from build123d import *

# Parameters (mm, degrees)
SKETCH_1_R          = 6
EXTRUDE_1_DEPTH     = 7.5
CUT_EXTRUDE_1_DEPTH = 26.75
SKETCH_4_W          = 4.5
SKETCH_4_H          = 2
CUT_EXTRUDE_2_DEPTH = 7
SKETCH_5_R          = 10
SKETCH_5_R_2        = 6
EXTRUDE_2_DEPTH     = 10
CHAMFER_1_SIZE      = 4
CHAMFER_2_SIZE      = 1
SKETCH_6_R          = 1.5
CUT_EXTRUDE_3_DEPTH = 61.309617807
SKETCH_8_R          = 2.5
CUT_EXTRUDE_4_DEPTH = 8
EXTRUDE_START       = 4
SKETCH_9_R          = 6
SKETCH_9_R_2        = 2.5
EXTRUDE_3_DEPTH     = 4
CHAMFER_4_SIZE      = 2


with BuildPart() as part:
    # 草图1 → 凸台-拉伸1 (new, symmetric)
    with BuildSketch(Plane.XY):
        with BuildLine():
            Line((-42.5, 16), (42.5, 16))
            ThreePointArc((42.5, 16), (49.571067812, 13.071067812), (52.5, 6))
            Line((52.5, 6), (52.5, -6))
            ThreePointArc((52.5, -6), (49.571067812, -13.071067812), (42.5, -16))
            Line((42.5, -16), (-42.5, -16))
            ThreePointArc((-42.5, -16), (-49.571067812, -13.071067812), (-52.5, -6))
            Line((-52.5, -6), (-52.5, 6))
            ThreePointArc((-52.5, 6), (-49.571067812, 13.071067812), (-42.5, 16))
        make_face()
        with Locations((-37.5, 0)):
            Circle(SKETCH_1_R, mode=Mode.SUBTRACT)
        with Locations((37.5, 0)):
            Circle(SKETCH_1_R, mode=Mode.SUBTRACT)
    extrude(amount=EXTRUDE_1_DEPTH, both=True)

    # 草图2 → 切除-拉伸1 (cut)
    with BuildSketch(Plane(origin=(0, 16, 0), x_dir=(1, 0, 0), z_dir=(0, 1, 0))):
        Polygon((13.15, 7.5), (11.35, 7.5), (11.35, 6.52), (9.29, 6.52), (9.29, 3.47), (11.35, 3.47), (11.35, 1.52), (9.29, 1.52), (9.29, -1.53), (11.35, -1.53), (11.35, -3.48), (9.29, -3.48), (9.29, -6.53), (11.35, -6.53), (11.35, -7.5), (13.15, -7.5), align=None)
    extrude(amount=-CUT_EXTRUDE_1_DEPTH, mode=Mode.SUBTRACT)

    # 草图4 → 切除-拉伸2 (cut)
    with BuildSketch(Plane(origin=(0, 16, 0), x_dir=(1, 0, 0), z_dir=(0, 1, 0))):
        with Locations((4.04, 4)):
            Rectangle(SKETCH_4_W, SKETCH_4_H)
        with Locations((4.04, 0)):
            Rectangle(SKETCH_4_W, SKETCH_4_H)
        with Locations((4.04, -4)):
            Rectangle(SKETCH_4_W, SKETCH_4_H)
        with Locations((18.4, 4)):
            Rectangle(SKETCH_4_W, SKETCH_4_H)
        with Locations((18.4, 0)):
            Rectangle(SKETCH_4_W, SKETCH_4_H)
        with Locations((18.4, -4)):
            Rectangle(SKETCH_4_W, SKETCH_4_H)
    extrude(amount=-CUT_EXTRUDE_2_DEPTH, mode=Mode.SUBTRACT)

    # 草图5 → 凸台-拉伸2 (add)
    # profile 1 of 2: a face of its own
    with BuildSketch(Plane.XY.offset(7.5)):
        with Locations(Location((-37.5, 0, 0), (0, 0, 180))):
            Circle(SKETCH_5_R)
        with Locations((-37.5, 0)):
            Circle(SKETCH_5_R_2, mode=Mode.SUBTRACT)
    # profile 2 of 2: a face of its own
    with BuildSketch(Plane.XY.offset(7.5)):
        with Locations(Location((37.5, 0, 0), (0, 0, 180))):
            Circle(SKETCH_5_R)
        with Locations((37.5, 0)):
            Circle(SKETCH_5_R_2, mode=Mode.SUBTRACT)
    extrude(amount=EXTRUDE_2_DEPTH)

    # 倒角1
    chamfer_1_edges = [part.edges().sort_by_distance(p)[0] for p in [
        (-27.5, 0, 7.5),
        (47.5, 0, 7.5),
    ]]
    chamfer(chamfer_1_edges, length=CHAMFER_1_SIZE)

    # 倒角2
    chamfer_2_edges = [part.edges().sort_by_distance(p)[0] for p in [
        (-43.5, 0, 17.5),
        (31.5, 0, 17.5),
    ]]
    chamfer(chamfer_2_edges, length=CHAMFER_2_SIZE)

    # 草图6 → 切除-拉伸3 (cut, through all)
    with BuildSketch(Plane(origin=(0, 0, -7.5), x_dir=(-1, 0, 0), z_dir=(0, 0, -1))):
        with Locations((0, 7.5)):
            Circle(SKETCH_6_R)
        with Locations((0, -7.5)):
            Circle(SKETCH_6_R)
    extrude(amount=-CUT_EXTRUDE_3_DEPTH, mode=Mode.SUBTRACT)

    # 草图8 → 切除-拉伸4 (cut)
    with BuildSketch(Plane.XY.offset(7.5)):
        with Locations((0, 7.5)):
            Circle(SKETCH_8_R)
        with Locations((0, -7.5)):
            Circle(SKETCH_8_R)
    extrude(amount=-CUT_EXTRUDE_4_DEPTH, mode=Mode.SUBTRACT)

    # 草图9 → 凸台-拉伸3 (add)
    # profile 1 of 2: a face of its own
    with BuildSketch(Plane.XY.offset(7.5).offset(EXTRUDE_START)):
        with Locations(Location((0, 7.5, 0), (0, 0, 180))):
            Circle(SKETCH_9_R)
        with Locations((0, 7.5)):
            Circle(SKETCH_9_R_2, mode=Mode.SUBTRACT)
    # profile 2 of 2: a face of its own
    with BuildSketch(Plane.XY.offset(7.5).offset(EXTRUDE_START)):
        with Locations(Location((0, -7.5, 0), (0, 0, 180))):
            Circle(SKETCH_9_R)
        with Locations((0, -7.5)):
            Circle(SKETCH_9_R_2, mode=Mode.SUBTRACT)
    extrude(amount=-EXTRUDE_3_DEPTH)

    # 倒角4
    chamfer_4_edges = [part.edges().sort_by_distance(p)[0] for p in [
        (6, 7.5, 11.5),
        (6, -7.5, 11.5),
    ]]
    chamfer(chamfer_4_edges, length=CHAMFER_4_SIZE)


solid = part.part
Model file for the job. Use its own axes, mm. A direction names the side the tool comes from. Give positions to 0.01 mm unless a question says otherwise; leave off trailing zeros. Loops run counter-clockwise (first coordinate to the right, second up) from the corner with the lowest first, then second, coordinate; pieces in that order, holes last.
1) Flat gauge pins, fed straight in: pin 1 Ø1.6 at (y, z) = (8.5, -3) entering from +X; pin 2 Ø2 at (x, z) = (5, -0.5) entering from +Y; pin 3 Ø6 at (x, z) = (40.5, 11.5) entering from +Y; pin 4 Ø1 at (y, z) = (-11, -0.5) entering from -X. Where does each tip first touch, or does it go through?
2) Tool access for faces 1 (the cylindrical face through (-0.54, -9.94, 5.58)), 2 (the flat face through (18, 13, -3)), 3 (the flat face through (-40, -7, 17.5)): list every direction of +Z, -Z, +X, -X, +Y, -Y with a clear straight run to the whole face (end or side of a thin tool).
3) Saw through at C-C (z = 14.5). Write the cut outline in (x, y).
4) Wall check: line 1 (Z direction, x = 18, y = 12); line 2 (Y direction, x = 0, z = 5.75); line 3 (Y direction, x = 0, z = -5.25). Give the ranges that are in metal, low to high.
5) Saw through at B-B (x = -37.5). Write the cut outline in (y, z), plus the area to 3 significant figures.
6) Pull direction Z, two halves, no side cores. Call faces 4 (the conical face through (-44, 0, 17)), 5 (the flat face through (16.15, 13, -4)), 6 (the flat face through (13.15, 3, 0)): +Z half, -Z half, draft (parallel to the pull), parting line (faces both ways), or undercut.
7) Saw through at A-A (x = 0). Count the separate pieces of the cut face and the enclosed holes in it, plus the area to 3 significant figures.
Answer block:
1. pin 1: stops at x = 52.35
1. pin 2: stops at y = 16
1. pin 3: stops at y = 12.72
1. pin 4: stops at x = -51.43
2. face 1: +Z
2. face 2: +Y
2. face 3: +Z, +X, -X, +Y, -Y
3. outline: circle Ø20 at (-37.5, 0); circle Ø20 at (37.5, 0); hole circle Ø12 at (-37.5, 0); hole circle Ø12 at (37.5, 0)
4. line 1: z = -7.5 to -5, -3 to -1, 1 to 3, 5 to 7.5
4. line 2: y = -16 to -10, -5 to 5, 10 to 16
4. line 3: y = -16 to -9, -6 to 6, 9 to 16
5. outline: (-16, -7.5) - (-6, -7.5) - (-6, 16.5) - (-7, 17.5) - (-10, 17.5) - (-10, 11.5) - (-14, 7.5) - (-16, 7.5) - close; (6, -7.5) - (16, -7.5) - (16, 7.5) - (14, 7.5) - (10, 11.5) - (10, 17.5) - (7, 17.5) - (6, 16.5) - close
5. area: 395 mm2
6. face 4: +Z half
6. face 5: undercut
6. face 6: draft
7. separate pieces: 3
7. enclosed holes: 0
7. area: 406 mm2
